from build123d import *

# Parameters (mm, degrees)
SKETCH_1_W          = 210
SKETCH_1_H          = 80
EXTRUDE_1_DEPTH     = 6
SKETCH_2_R          = 2
CUT_EXTRUDE_1_DEPTH = 6
SKETCH_3_R          = 2
CUT_EXTRUDE_2_DEPTH = 20
SKETCH_4_R          = 3.3
CUT_EXTRUDE_3_DEPTH = 10
SKETCH_5_R          = 3.3
CUT_EXTRUDE_4_DEPTH = 10


with BuildPart() as part:
    # 草图1 → 凸台-拉伸1 (new body)
    with BuildSketch(Plane.XY):
        Rectangle(SKETCH_1_W, SKETCH_1_H)
    extrude(amount=EXTRUDE_1_DEPTH)

    # 草图2 → 切除-拉伸1 (cut)
    with BuildSketch(Plane.XY.offset(6)):
        with Locations((-102, 0)):
            Circle(SKETCH_2_R)
        with Locations((-102, 37)):
            Circle(SKETCH_2_R)
        with Locations((-102, -37)):
            Circle(SKETCH_2_R)
        with Locations((-34, 37)):
            Circle(SKETCH_2_R)
        with Locations((34, 37)):
            Circle(SKETCH_2_R)
        with Locations((102, 37)):
            Circle(SKETCH_2_R)
    extrude(amount=-CUT_EXTRUDE_1_DEPTH, mode=Mode.SUBTRACT)

    # 草图3 → 切除-拉伸2 (cut)
    with BuildSketch(Plane(origin=(105, 0, 0), x_dir=(0, 0, -1), z_dir=(1, 0, 0))):
        with Locations((-3, -37)):
            Circle(SKETCH_3_R)
        with Locations((-3, 13)):
            Circle(SKETCH_3_R)
    extrude(amount=-CUT_EXTRUDE_2_DEPTH, mode=Mode.SUBTRACT)

    # 草图4 → 切除-拉伸3 (cut)
    with BuildSketch(Plane.XY.offset(6)):
        with Locations((-86, 10)):
            Circle(SKETCH_4_R)
        with Locations((-86, -10)):
            Circle(SKETCH_4_R)
    extrude(amount=-CUT_EXTRUDE_3_DEPTH, mode=Mode.SUBTRACT)

    # 草图5 → 切除-拉伸4 (cut)
    with BuildSketch(Plane.XY.offset(6)):
        with Locations((-42, 21)):
            Circle(SKETCH_5_R)
        with Locations((-22, 21)):
            Circle(SKETCH_5_R)
    extrude(amount=-CUT_EXTRUDE_4_DEPTH, mode=Mode.SUBTRACT)


solid = part.part
Source: CAD feature listing. Evaluate the final solid. Frame: model axes, mm. A direction names the side the tool comes from. Give positions to 0.01 mm unless a question says otherwise; leave off trailing zeros. Write each loop counter-clockwise with the first axis right and the second up, starting at its lowest first coordinate (ties: lowest second). Pieces come first, ordered by that corner, then holes. Notation, with made-up numbers: M 6.5,4 L 64.5,4 A13 cw 64.5,26 Z; hole C -27.5,47.5 d7. An arc over 180 degrees is marked long. Answer as a JSON object with one key per item and string values.
Q1. Cut plane D-D, the plane z = 2.5. Count the separate pieces of the cut face and the enclosed holes in it, then the cut area to 3 significant figures.
Geometry check:
{"separate pieces": "1", "enclosed holes": "10", "area": "16,400 mm^2"}
Q2. Mould query, pull axis Y, two halves, no side actions, for faces 3 (the face through (-105, -1, 3)), 4 (the face through (85, 13, 3)), 5 (the face through (-1, -40, 3)). Classes: +Y half, -Y half, draft (parallel to the pull), parting line (faces both ways), or undercut.
Geometry check:
{"face 3": "draft", "face 4": "undercut", "face 5": "-Y half"}
Q3. Ray query, line 1 along Y through (x, z) = (-86, 2.85); line 2 along Y through (x, z) = (-102, 3.2); line 3 along Y through (x, z) = (-22, 3.1). Return the intervals inside material, ascending.
Geometry check:
{"line 1": "y = -40 to -13.3, -6.7 to 6.7, 13.3 to 40", "line 2": "y = -40 to -39, -35 to -2, 2 to 35, 39 to 40", "line 3": "y = -40 to 17.7, 24.3 to 40"}
Q4. Cut plane A-A, the plane y = 21. Return the cut outline in (x, z).
Geometry check:
{"outline": "M -105,0 L -45.3,0 L -45.3,6 L -105,6 Z; M -38.7,0 L -25.3,0 L -25.3,6 L -38.7,6 Z; M -18.7,0 L 105,0 L 105,6 L -18.7,6 Z"}
Q5. Cut plane B-B, the plane x = -22. Return the cut outline in (y, z), then the cut area to 3 significant figures.
Geometry check:
{"outline": "M -40,0 L 17.7,0 L 17.7,6 L -40,6 Z; M 24.3,0 L 40,0 L 40,6 L 24.3,6 Z", "area": "440 mm^2"}
Q6. Access query for faces 1 (the face through (95, -39, 3)), 2 (the face through (-1, 40, 3)). Directions: +Z, -Z, +X, -X, +Y, -Y. A direction counts if a zero-diameter tool reaches every point of the face in a straight line with its end or side. Return the directions, or none.
Geometry check:
{"face 1": "+X", "face 2": "+Z, -Z, +X, -X, +Y"}
Q7. Cut plane C-C, the plane y = 0. Return the cut outline in (x, z), then the cut area to 3 significant figures.
Geometry check:
{"outline": "M -105,0 L -104,0 L -104,6 L -105,6 Z; M -100,0 L 105,0 L 105,6 L -100,6 Z", "area": "1,240 mm^2"}
